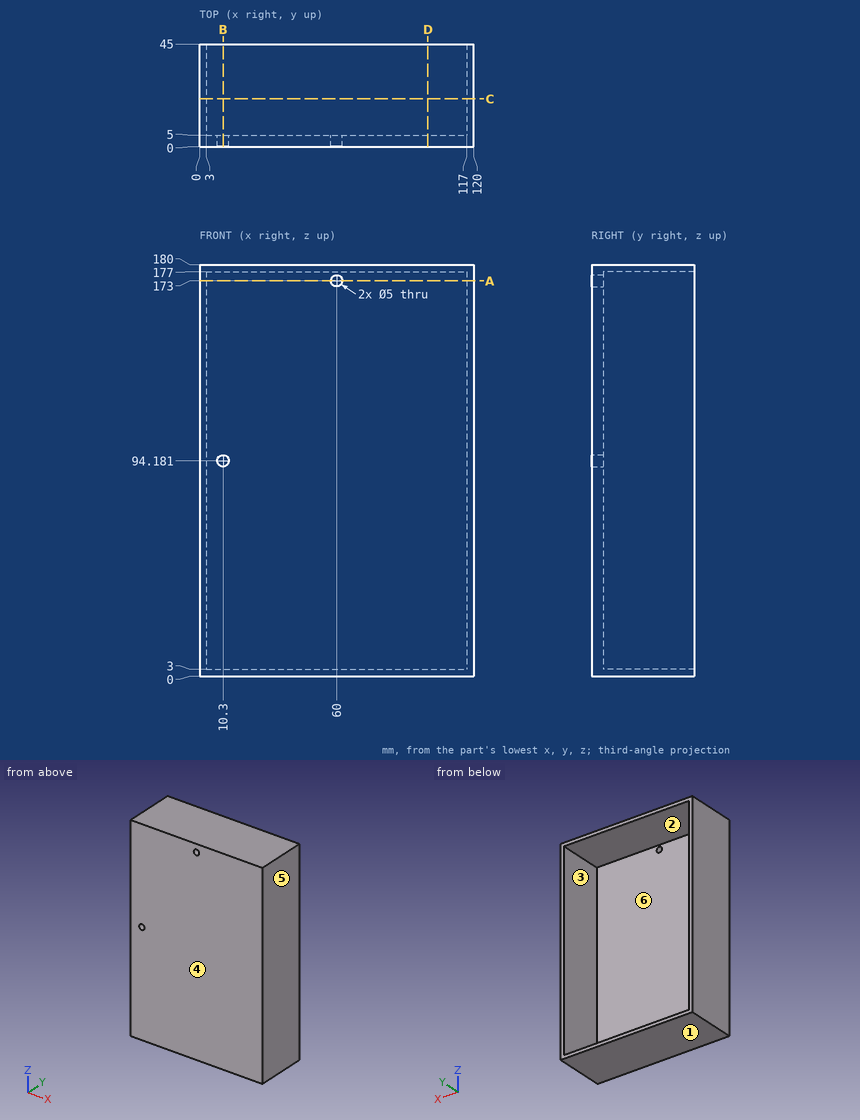
Study the drawing (mm; zero at the part's minimum x, y, z) and answer. A direction names the side the tool comes from. Coordinates: 2 decimals unless noted, no trailing zeros. Order: outer loops, then holes, each group sorted by start corner. A loop starts at its lowest first (then second) coordinate and runs counter-clockwise, first axis right, second up. Notation, with made-up numbers: M 37,65.25 L 73,65.25 A17 ccw 73,84.25 Z; hole C 36.5,41.25 d11. An arc over 180 degrees is marked long. Use CSV: the item, a comma, the result in double quotes.
Q1. Section A-A (z = 173) is taken. Determine the outline of the cut face in (x, y).
Here are the results:
outline,"M 0,0 L 57.5,0 L 57.5,5 L 3,5 L 3,45 L 0,45 Z; M 62.5,0 L 120,0 L 120,45 L 117,45 L 117,5 L 62.5,5 Z"
Q2. Section D-D (x = 100) is taken. Determine the outline of the cut face in (y, z), then the cut area to 3 significant figures.
Here are the results:
outline,"M 0,0 L 45,0 L 45,3 L 5,3 L 5,177 L 45,177 L 45,180 L 0,180 Z"
area,"1,140 mm2"
Q3. Section C-C (y = 21) is taken. Determine the outline of the cut face in (x, z).
Here are the results:
outline,"M 0,0 L 120,0 L 120,180 L 0,180 Z; hole M 3,3 L 117,3 L 117,177 L 3,177 Z"
Q4. Given pin 1 Ø4.5 at (x, z) = (10.3, 94.18) entering from -Y; pin 2 Ø12 at (x, z) = (92, 100.5) entering from +Y, each flat-ended and moving along its own axis, determine where each tip first touches the part or whether it passes through.
Here are the results:
pin 1,"through"
pin 2,"y = 5"
Q5. A tool of negligible diameter and unlimited length cuts with its end or side. For the marked faces 5 and 6, from which of +Z, -Z, +X, -X, +Y, -Y can it reach the whole face along a straight path? Write none if from no direction.
Here are the results:
face 5,"+Z, -Z, +X, +Y, -Y"
face 6,"+Y"
Q6. Section B-B (x = 10.3) is taken. Determine the outline of the cut face in (y, z).
Here are the results:
outline,"M 0,0 L 45,0 L 45,3 L 5,3 L 5,91.68 L 0,91.68 Z; M 0,96.68 L 5,96.68 L 5,177 L 45,177 L 45,180 L 0,180 Z"
Q7. Determine the mould class of the marked faces 1, 2, 3 and 4 for opening direction Z: pulls with the +Z half, pulls with the -Z half, needs draft (parallel to the pull), parting line crosses it, or undercut.
Here are the results:
face 1,"pulls with the -Z half"
face 2,"undercut"
face 3,"undercut"
face 4,"needs draft"
Q8. Straight lines are drawn through the part: L1, parallel to Z at x = 33, y = 16.5; L2, parallel to X at y = 31, z = 141; L3, parallel to X at y = 2, z = 173. For each, find the intervals that lie inside material, in ascending order.
Here are the results:
L1,"0 to 3, 177 to 180"
L2,"0 to 3, 117 to 120"
L3,"0 to 57.5, 62.5 to 120"
